Can you work these out from the drawing? Everything is in mm from the part's minimum corner. A direction names the side the tool comes from. Coordinates: 2 decimals unless noted, no trailing zeros. Order: outer loops, then holes, each group sorted by start corner. A loop starts at its lowest first (then second) coordinate and runs counter-clockwise, first axis right, second up. Notation, with made-up numbers: (63.25, -27.5) -> (87.25, -27.5) arc R30 ccw to (87.25, 5.5) -> close; hole circle Ø2 at (68.5, -16.75). An arc over 180 degrees is marked (long way). Put each result on its own line as item: value. Start each with the question number.
Q1. Please list where these lines run through material, in increasing order: line 1 along X through (y, z) = (10.5, 35); line 2 along Y through (x, z) = (33, 27); line 3 along X through (y, z) = (13.5, 30).
Q2. We'd pull the mould along Z, two halves only. Please class the marked faces 1, 2 and 3: +Z half, -Z half, draft (parallel to the pull), parting line (faces both ways), or undercut.
Q3. Will these pins go through, and if not, where does the flat tip stop? pin 1 (3 mm diameter, centred on y = 3, z = 16, fed in from +X); pin 2 (6 mm diameter, centred on x = 27.5, y = 7, fed in from +Z); pin 3 (1.5 mm diameter, centred on x = 62.5, y = 11, fed in from +Z).
Q4. If we section it at B-B (x = 35): Please give me the cut outline in (y, z).
Q5. For the marked faces 4 and 5, which set-ups out of +Z, -Z, +X, -X, +Y, -Y let a thin tool reach every point of the face, with its end or its side?
Q6. If we section it at C-C (y = 6): Please give me the cut outline in (x, z).
Q7. If we section it at A-A (z = 35): Please give me the cut outline in (x, y).
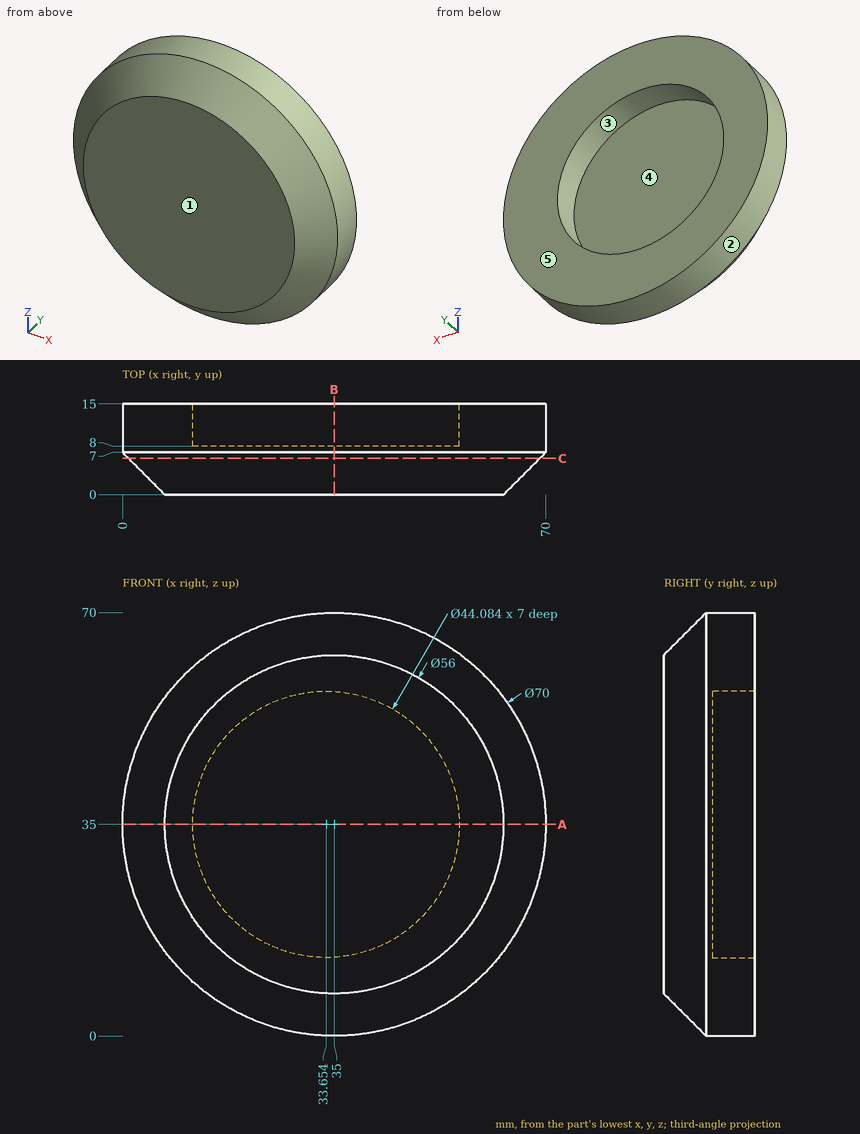
The answers:
1. line 1: 0 to 11.61, 55.7 to 70
1. line 2: 0 to 8
1. line 3: 0.36 to 12.19, 55.12 to 69.64
2. face 1: draft
2. face 2: parting line
2. face 3: undercut
3. pin 1: x = 61.65
3. pin 2: z = 69.71
3. pin 3: z = 57.57
4. outline: (0, 7) -> (7, 0) -> (15, 0) -> (15, 13) -> (8, 13) -> (8, 57) -> (15, 57) -> (15, 70) -> (7, 70) -> (0, 63) -> close
5. face 4: +Y
5. face 5: +Z, -Z, +X, -X, +Y
6. outline: circle Ø68 at (35, 35)
7. outline: (0, 7) -> (7, 0) -> (63, 0) -> (70, 7) -> (70, 15) -> (55.7, 15) -> (55.7, 8) -> (11.61, 8) -> (11.61, 15) -> (0, 15) -> close
